Source: CAD feature listing. Evaluate the final solid. Frame: model axes, mm. Face numbers are marked on the shaded views. A direction names the side the tool comes from. Coordinates: 2 decimals unless noted, no trailing zeros. Loops run counter-clockwise (first coordinate to the right, second up) from the corner with the lowest first, then second, coordinate; pieces in that order, holes last.
```python
from build123d import *

# Parameters (mm, degrees)
SKETCH1_W           = 30
SKETCH1_H           = 16
BOSS_EXTRUDE1_DEPTH = 3
SKETCH2_W           = 3
SKETCH2_H           = 16
BOSS_EXTRUDE2_DEPTH = 5.4
SKETCH3_R           = 1.5
CUT_EXTRUDE1_DEPTH  = 5.4
SKETCH4_R           = 1.5
CUT_EXTRUDE2_DEPTH  = 10


with BuildPart() as part:
    # Sketch1 → Boss-Extrude1 (new body)
    with BuildSketch(Plane(origin=(0, 0, 0), x_dir=(1, 0, 0), z_dir=(0, 1, 0))):
        Rectangle(SKETCH1_W, SKETCH1_H)
    extrude(amount=BOSS_EXTRUDE1_DEPTH)

    # Sketch2 → Boss-Extrude2 (add)
    with BuildSketch(Plane(origin=(0, 3, 0), x_dir=(1, 0, 0), z_dir=(0, 1, 0))):
        with Locations((-13.5, 0)):
            Rectangle(SKETCH2_W, SKETCH2_H)
    boss_extrude2 = extrude(amount=BOSS_EXTRUDE2_DEPTH)

    # Sketch3 → Cut-Extrude1 (cut)
    with BuildSketch(Plane.ZY.offset(15)):
        with Locations((-4, 5.4)):
            Circle(SKETCH3_R)
        with Locations((4, 5.4)):
            Circle(SKETCH3_R)
    cut_extrude1 = extrude(amount=-CUT_EXTRUDE1_DEPTH, mode=Mode.SUBTRACT)

    # Mirror1: Boss-Extrude2, Cut-Extrude1 across plane
    add(boss_extrude2.mirror(Plane(origin=(0, 0, 0), x_dir=(0, 0, 1), z_dir=(1, 0, 0))))
    add(cut_extrude1.mirror(Plane(origin=(0, 0, 0), x_dir=(0, 0, 1), z_dir=(1, 0, 0))), mode=Mode.SUBTRACT)

    # Sketch4 → Cut-Extrude2 (cut)
    with BuildSketch(Plane(origin=(0, 3, 0), x_dir=(1, 0, 0), z_dir=(0, 1, 0))):
        Circle(SKETCH4_R)
    extrude(amount=-CUT_EXTRUDE2_DEPTH, mode=Mode.SUBTRACT)


solid = part.part
```
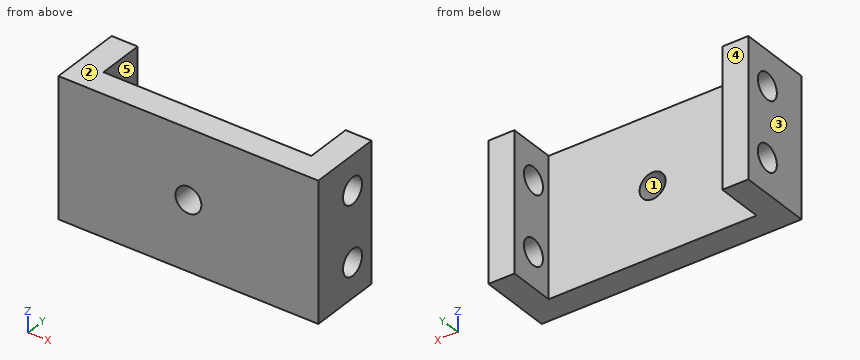
Q1. Reachability of the marked faces 4 and 5 from +Z, -Z, +X, -X, +Y, -Y: full face, straight path, thin tool, end or side. Return the list, or none.
Q2. Draft query along X for the marked faces 1, 2 and 3. Return one class per face: released by +X, released by -X, zero draft, split by the parting line, or undercut.
Q3. Section query C-C on z = 0. Return the cut outline in (x, y).
Q4. Section query D-D on z = 7. Return the cut outline in (x, y), then the cut area to 3 significant figures.
Q5. Section query A-A on z = 4. Return the cut outline in (x, y), then the cut area to 3 significant figures.
Q6. Material intervals for line 1 along Y through (x, z) = (-12.55, 4); line 2 along X through (y, z) = (4.25, 7); line 3 along Z through (x, y) = (0, 1.8), sorted ascending.
Q7. Section query B-B on y = 7.75. Return the cut outline in (x, z), then the cut area to 3 significant figures.
Q8. First-contact query: pin 1 Ø2.5 at (y, z) = (5.4, -4) entering from -X; pin 2 Ø2 at (x, y) = (-7.5, 3.5) entering from +Z; pin 3 Ø6 at (x, z) = (6.5, 6) entering from +Y. Flat tips, straight axial feed; report the tip coordinate or a pass-through.
Resolved:
1. face 4: +Z, -Z, +X, -X, +Y
1. face 5: +Z, -Z, +Y
2. face 1: undercut
2. face 2: zero draft
2. face 3: released by -X
3. outline: (-15, 0) - (-1.5, 0) - (-1.5, 3) - (-12, 3) - (-12, 8.4) - (-15, 8.4) - close; (1.5, 0) - (15, 0) - (15, 8.4) - (12, 8.4) - (12, 3) - (1.5, 3) - close
4. outline: (-15, 0) - (15, 0) - (15, 8.4) - (12, 8.4) - (12, 3) - (-12, 3) - (-12, 8.4) - (-15, 8.4) - close
4. area: 122 mm2
5. outline: (-15, 0) - (15, 0) - (15, 3.9) - (12, 3.9) - (12, 3) - (-12, 3) - (-12, 3.9) - (-15, 3.9) - close; (-15, 6.9) - (-12, 6.9) - (-12, 8.4) - (-15, 8.4) - close; (12, 6.9) - (15, 6.9) - (15, 8.4) - (12, 8.4) - close
5. area: 104 mm2
6. line 1: y = 0 to 3.9, 6.9 to 8.4
6. line 2: x = -15 to -12, 12 to 15
6. line 3: z = -8 to -1.5, 1.5 to 8
7. outline: (-15, -8) - (-12, -8) - (-12, 8) - (-15, 8) - close; (12, -8) - (15, -8) - (15, 8) - (12, 8) - close
7. area: 96.0 mm2
8. pin 1: passes through
8. pin 2: stops at z = 8
8. pin 3: stops at y = 3
